Here's how the part is built. I have some questions about the finished solid (model axes, mm). A direction names the side the tool comes from. Round coordinates to 2 decimals unless told otherwise and drop trailing zeros. Loops run counter-clockwise (first coordinate to the right, second up) from the corner with the lowest first, then second, coordinate; pieces in that order, holes last. Notation, with made-up numbers: M 45.5,76 L 81.5,76 A18 ccw 81.5,82 Z; hole C 34,-9.5 d7. An arc over 180 degrees is marked long. One line per question, with ' | ' between items. Start each with the question number.
```python
from build123d import *

# Parameters (mm, degrees)
SKETCH_10_R     = 1
EXTRUDE_5_DEPTH = 5
EXTRUDE_START   = 2
SKETCH_10_4_W   = 97.99999928
SKETCH_10_4_H   = 16.500549096
SKETCH_10_4_R   = 1
EXTRUDE_6_DEPTH = 2
EXTRUDE_START_2 = 4
SKETCH_11_R     = 2
SKETCH_11_R_2   = 1
EXTRUDE_8_DEPTH = 4
FILLET_30_R     = 3


with BuildPart() as part:
    # Sketch 10 → Extrude 5 (new body)
    with BuildSketch(Plane(origin=(0, 10, 0), x_dir=(1, 0, 0), z_dir=(0, 1, 0))):
        Polygon((8.00000036, 17.5), (-3.99999964, 17.5), (-3.99999964, 12.999450904), (93.99999964, 12.999450904), (93.99999964, 17.5), (81.99999964, 17.5), (81.99999964, 29.5), (8.00000036, 29.5), align=None)
        with Locations(Location((16.003399367, 18.999450904, 0), (0, 0, 270))):
            Circle(SKETCH_10_R, mode=Mode.SUBTRACT)
        with Locations(Location((74.003399367, 18.999450904, 0), (0, 0, 270))):
            Circle(SKETCH_10_R, mode=Mode.SUBTRACT)
    extrude(amount=-EXTRUDE_5_DEPTH)

    # Sketch 10_4 → Extrude 6 (add)
    with BuildSketch(Plane(origin=(0, 10, 0), x_dir=(1, 0, 0), z_dir=(0, 1, 0)).offset(EXTRUDE_START)):
        with Locations((45, 21.249725452)):
            Rectangle(SKETCH_10_4_W, SKETCH_10_4_H)
        with Locations(Location((2.00000036, 23.5, 0), (0, 0, 270))):
            Circle(SKETCH_10_4_R, mode=Mode.SUBTRACT)
        with Locations(Location((88.00000036, 23.5, 0), (0, 0, 270))):
            Circle(SKETCH_10_4_R, mode=Mode.SUBTRACT)
        with Locations(Location((16.003399367, 18.999450904, 0), (0, 0, 270))):
            Circle(SKETCH_10_4_R, mode=Mode.SUBTRACT)
        with Locations(Location((74.003399367, 18.999450904, 0), (0, 0, 270))):
            Circle(SKETCH_10_4_R, mode=Mode.SUBTRACT)
    extrude(amount=-EXTRUDE_6_DEPTH)

    # Sketch 11 → Extrude 8 (add)
    # profile 1 of 2: a face of its own
    with BuildSketch(Plane(origin=(0, 12, 0), x_dir=(1, 0, 0), z_dir=(0, 1, 0)).offset(EXTRUDE_START_2)):
        with Locations(Location((16.003399367, 18.999450904, 0), (0, 0, 270))):
            Circle(SKETCH_11_R)
        with Locations(Location((16.003399367, 18.999450904, 0), (0, 0, 270))):
            Circle(SKETCH_11_R_2, mode=Mode.SUBTRACT)
    # profile 2 of 2: a face of its own
    with BuildSketch(Plane(origin=(0, 12, 0), x_dir=(1, 0, 0), z_dir=(0, 1, 0)).offset(EXTRUDE_START_2)):
        with Locations(Location((74.003399367, 18.999450904, 0), (0, 0, 270))):
            Circle(SKETCH_11_R)
        with Locations(Location((74.003399367, 18.999450904, 0), (0, 0, 270))):
            Circle(SKETCH_11_R_2, mode=Mode.SUBTRACT)
    extrude(amount=-EXTRUDE_8_DEPTH)

    # Fillet 30
    fillet_30_edges = [part.edges().sort_by_distance(p)[0] for p in [
        (16.003399367, 12, -20.999450904),
        (74.003399367, 12, -20.999450904),
    ]]
    fillet(fillet_30_edges, radius=FILLET_30_R)


solid = part.part
```
1) We'd pull the mould along X, two halves only. Please class faces 1 (the face through (14.05, 15.51, -19.43)), 2 (the face through (8, 8, -24)), 3 (the face through (44, 9, -12.999)): pulls with the +X half, pulls with the -X half, needs draft (parallel to the pull), parting line crosses it, or undercut.
2) Imagine slicing it at C-C (z = -25.5). Write out the boundary of the cut face in (x, y), then the cut area to 3 significant figures.
3) For faces 4 (the face through (82, 8, -23)), 5 (the face through (72.05, 15.51, -19.43)), 6 (the face through (2, 8, -17.5)), which set-ups out of +Z, -Z, +X, -X, +Y, -Y let a thin tool reach every point of the face, with its end or its side?
4) Imagine slicing it at B-B (y = 8.5). Write out the boundary of the cut face in (x, z).
5) Imagine slicing it at A-A (x = 2). Write out the boundary of the cut face in (y, z).
6) I'm going to push flat-ended pins straight in: pin 1 Ø1.8 at (x, z) = (2, -23.5) entering from -Y; pin 2 Ø3.5 at (x, z) = (2, -24.5) entering from -Y; pin 3 Ø4 at (x, y) = (88, 7) entering from -Z; pin 4 Ø4 at (y, z) = (7.5, -21) entering from +X. Where does each tip first touch, or does it pass through?
7) Imagine slicing it at D-D (x = 63). Write out the boundary of the cut face in (y, z), then the cut area to 3 significant figures.
8) Please list where these lines run through material, in increasing order: L1, parallel to X at y = 9.5, z = -19; L2, parallel to X at y = 11, z = -23.5; L3, parallel to Y at x = 22.5, z = -15. Write a range as from..to.
Results are:
1) face 1: undercut | face 2: pulls with the -X half | face 3: needs draft
2) outline: M -4,10 L 8,10 L 8,5 L 82,5 L 82,10 L 94,10 L 94,12 L -4,12 Z | area: 566 mm²
3) face 4: -Z, +X, -Y | face 5: +Y | face 6: -Z, -X, -Y
4) outline: M -4,-17.5 L 8,-17.5 L 8,-29.5 L 82,-29.5 L 82,-17.5 L 94,-17.5 L 94,-13 L -4,-13 Z; hole C 16,-19 d2; hole C 74,-19 d2
5) outline: M 5,-17.5 L 10,-17.5 L 10,-22.5 L 12,-22.5 L 12,-13 L 5,-13 Z; M 10,-29.5 L 12,-29.5 L 12,-24.5 L 10,-24.5 Z
6) pin 1: through | pin 2: y = 10 | pin 3: z = -17.5 | pin 4: x = 82
7) outline: M 5,-29.5 L 12,-29.5 L 12,-13 L 5,-13 Z | area: 116 mm²
8) L1: 8..15, 17..73, 75..82 | L2: -4..1, 3..87, 89..94 | L3: 5..12
